from build123d import *

# Parameters (mm, degrees)
F1_DEPTH = 3.175
F2_W     = 0.8128
F2_H     = 18.520833
F2_H_2   = 18.520834
F2_W_2   = 9.071428
F2_H_3   = 0.8128
F3_DEPTH = 0.8128


with BuildPart() as f1:
    # F0 (on Top) → F1 (new body)
    with BuildSketch(Plane.XY):
        Polygon((0, 111.125), (0, 187.325), (-25.4, 187.325), (-25.4, 142.875), (-38.1, 142.875), (-38.1, 187.325), (-63.5, 187.325), (-63.5, 111.125), (-139.7, 111.125), (-139.7, 0), (-63.5, 0), (-63.5, -76.2), (-38.1, -76.2), (-38.1, -31.75), (-25.4, -31.75), (-25.4, -76.2), (0, -76.2), (0, 0), (220.98, 0), (220.98, 111.125), align=None)
    extrude(amount=F1_DEPTH)

    # F2 (on face) → F3 (join)
    with BuildSketch(Plane.XY.offset(3.175)):
        with Locations((-63.9064, 101.864583)):
            Rectangle(F2_W, F2_H)
        with Locations((-63.9064, 64.822916)):
            Rectangle(F2_W, F2_H)
        with Locations((-63.9064, 27.78125)):
            Rectangle(F2_W, F2_H_2)
        with Locations((0.4064, 27.78125)):
            Rectangle(F2_W, F2_H_2)
        with Locations((0.4064, 64.822916)):
            Rectangle(F2_W, F2_H)
        with Locations((0.4064, 101.864583)):
            Rectangle(F2_W, F2_H)
        with Locations((76.6064, 101.889292)):
            Rectangle(F2_W, F2_H_2)
        with Locations((76.6064, 64.847625)):
            Rectangle(F2_W, F2_H)
        with Locations((76.6064, 27.547179)):
            Rectangle(F2_W, F2_H)
        with Locations((140.1064, 101.864583)):
            Rectangle(F2_W, F2_H)
        with Locations((140.1064, 27.52247)):
            Rectangle(F2_W, F2_H)
        with Locations((140.1064, 64.822916)):
            Rectangle(F2_W, F2_H)
        with Locations((148.0439, 101.864583)):
            Rectangle(F2_W, F2_H)
        with Locations((148.0439, 64.822916)):
            Rectangle(F2_W, F2_H)
        with Locations((148.0439, 27.78125)):
            Rectangle(F2_W, F2_H_2)
        with Locations((-49.892857, -0.4064)):
            Rectangle(F2_W_2, F2_H_3)
        with Locations((-31.75, -0.4064)):
            Rectangle(F2_W_2, F2_H_3)
        with Locations((-13.607143, -0.4064)):
            Rectangle(F2_W_2, F2_H_3)
        with Locations((-31.75, 111.5314)):
            Rectangle(F2_W_2, F2_H_3)
        with Locations((-13.607143, 111.5314)):
            Rectangle(F2_W_2, F2_H_3)
        with Locations((-49.892857, 111.5314)):
            Rectangle(F2_W_2, F2_H_3)
    extrude(amount=F3_DEPTH)


solid = f1.part
Geometry check sheet. Reference: the model listing, model coordinates, mm. Round coordinates to 2 decimals unless told otherwise and drop trailing zeros. Write each loop counter-clockwise with the first axis right and the second up, starting at its lowest first coordinate (ties: lowest second). Pieces come first, ordered by that corner, then holes.
Item 1: Section check D-D (y = -17). Record the boundary of the cut face in (x, z) (3 decimals), plus the area to 3 significant figures.
Determined:
outline: (-63.5, 0) - (0, 0) - (0, 3.175) - (-63.5, 3.175) - close
area: 202 mm2
Item 2: Mould release check, pull along X, two halves, no side actions. Record for faces 1 (the face through (38, 57, 3.175)), 2 (the face through (38, 57, 0)): +X half, -X half, draft (parallel to the pull), parting line (faces both ways), or undercut.
Determined:
face 1: undercut
face 2: draft
Item 3: Material ranges on line 1 along X through (y, z) = (63.5, 3.25); line 2 along X through (y, z) = (-34, 2.45); line 3 along Y through (x, z) = (47, 0.2) (3 decimals), recorded low to high.
Determined:
line 1: x = -64.31 to -63.5, 0 to 0.81, 76.2 to 77.01, 139.7 to 140.51, 147.64 to 148.45
line 2: x = -63.5 to -38.1, -25.4 to 0
line 3: y = 0 to 111.125
Item 4: Section check B-B (z = 0.75). Record the boundary of the cut face in (x, y) (3 decimals).
Determined:
outline: (-139.7, 0) - (-63.5, 0) - (-63.5, -76.2) - (-38.1, -76.2) - (-38.1, -31.75) - (-25.4, -31.75) - (-25.4, -76.2) - (0, -76.2) - (0, 0) - (220.98, 0) - (220.98, 111.125) - (0, 111.125) - (0, 187.325) - (-25.4, 187.325) - (-25.4, 142.875) - (-38.1, 142.875) - (-38.1, 187.325) - (-63.5, 187.325) - (-63.5, 111.125) - (-139.7, 111.125) - close
Item 5: Section check A-A (y = 154). Record the boundary of the cut face in (x, z) (3 decimals), plus the area to 3 significant figures.
Determined:
outline: (-63.5, 0) - (-38.1, 0) - (-38.1, 3.175) - (-63.5, 3.175) - close; (-25.4, 0) - (0, 0) - (0, 3.175) - (-25.4, 3.175) - close
area: 161 mm2
Item 6: Section check C-C (x = 28.5). Record the boundary of the cut face in (y, z) (3 decimals).
Determined:
outline: (0, 0) - (111.125, 0) - (111.125, 3.175) - (0, 3.175) - close
Item 7: Go/stop test with flat-tipped pins: pin 1 Ø1.6 at (y, z) = (-43.5, 1) entering from +X; pin 2 Ø0.9 at (x, z) = (148, 3.5) entering from -Y; pin 3 Ø0.7 at (x, z) = (148, 3.5) entering from +Y (3 decimals). Record where each tip stops, or that it passes through.
Determined:
pin 1: stops at x = 0
pin 2: stops at y = 0
pin 3: stops at y = 111.125
